Could you check a few things on this model? Use its own coordinates, in mm. Face numbers are marked on the shaded views. A direction names the side the tool comes from. Coordinates: 2 decimals unless noted, no trailing zeros. Loops run counter-clockwise (first coordinate to the right, second up) from the corner with the lowest first, then second, coordinate; pieces in that order, holes last.
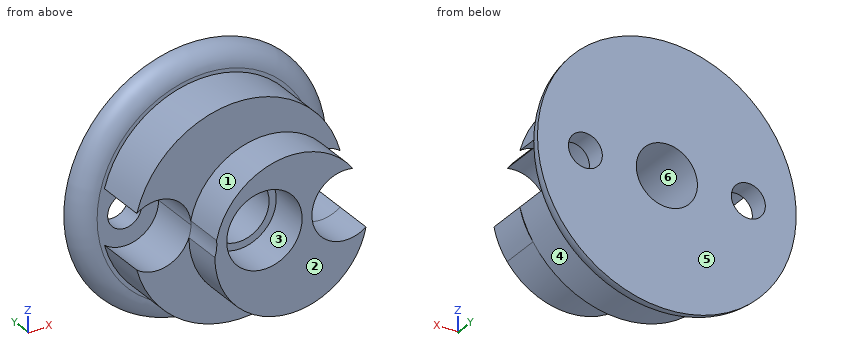
from build123d import *

# Parameters (mm, degrees)
F0_R     = 19.05
F0_R_2   = 2.5
F0_R_3   = 4.5
F1_DEPTH = 3
F2_R     = 2.99999
F3_R     = 4.5
F4_DEPTH = 7.5
F5_R     = 5.555
F6_DEPTH = 6


# Not quite as in the source:
# - a fillet or chamfer is up to 0.001 mm smaller than in the source, because OpenCascade refuses the exact size


with BuildPart() as f1:
    # F0 (on Front) → F1 (new body)
    with BuildSketch(Plane.XZ):
        Circle(F0_R)
        with Locations((-12, 0)):
            Circle(F0_R_2, mode=Mode.SUBTRACT)
        Circle(F0_R_3, mode=Mode.SUBTRACT)
        with Locations((12, 0)):
            Circle(F0_R_2, mode=Mode.SUBTRACT)
    extrude(amount=F1_DEPTH)

    # F2 (radius 3 in the source; OpenCascade refuses exactly that, so slightly less here)
    f2_edges = [f1.edges().sort_by_distance(p)[0] for p in [
        (-19.05, -3, 0),
    ]]
    fillet(f2_edges, radius=F2_R)

    # F3 (on face) → F4 (join)
    with BuildSketch(Plane.XZ.offset(3)):
        with BuildLine():
            ThreePointArc((14.96875, -4.0232478717), (7, 0), (14.96875, 4.0232478717))
            ThreePointArc((14.96875, 4.0232478717), (0, 15.5), (-14.96875, 4.0232478717))
            ThreePointArc((-14.96875, 4.0232478717), (-9.7465304528, 4.4633927678), (-7, 0))
            ThreePointArc((-7, 0), (-9.7465304528, -4.4633927678), (-14.96875, -4.0232478717))
            ThreePointArc((-14.96875, -4.0232478717), (0, -15.5), (14.96875, -4.0232478717))
        make_face()
        Circle(F3_R, mode=Mode.SUBTRACT)
    extrude(amount=F4_DEPTH)

    # F5 (on face) → F6 (join)
    with BuildSketch(Plane.XZ.offset(10.5)):
        with BuildLine():
            ThreePointArc((13.0379586998, -8.3822212416), (14.2369080678, -6.3061863212), (14.96875, -4.0232478717))
            ThreePointArc((14.96875, -4.0232478717), (14.1719474758, -6.2774122648), (13.0379586998, -8.3822212416))
        make_face()
        with BuildLine():
            ThreePointArc((13.0379586998, -8.3822212416), (14.1719474758, -6.2774122648), (14.96875, -4.0232478717))
            ThreePointArc((14.96875, -4.0232478717), (7.1141405648, -1.0622511849), (13.0303045981, 4.8926958249))
            ThreePointArc((13.0303045981, 4.8926958249), (1.6209007027, 9.2560887381), (-7.0415959869, 0.6436067458))
            ThreePointArc((-7.0415959869, 0.6436067458), (-7.0298229821, -0.5452892911), (-7.2990861299, -1.7033522202))
            ThreePointArc((-7.2990861299, -1.7033522202), (0.4406594059, -12.4383718384), (13.0379586998, -8.3822212416))
        make_face()
        Circle(F5_R, mode=Mode.SUBTRACT)
    extrude(amount=F6_DEPTH)


solid = f1.part
1) Imagine slicing it at A-A on y = -10. List the corners of the cut face in (x, z) for me.
2) Imagine slicing it at C-C on y = -1.75. List the corners of the cut face in (x, z) for me.
3) We'd pull the mould along Z, two halves only. Please class the marked faces 4, 5 and 6: released by +Z, released by -Z, zero draft, split by the parting line, or undercut.
4) If I drill on L1, parallel to Y at x = -1, z = -13.5; L2, parallel to Z at x = 12, y = -11.75; L3, parallel to Z at x = 12, y = -0.85, over which ranges is the centre line in solid material (lowest first)?
5) For the marked faces 1, 2 and 3, which set-ups out of +Z, -Z, +X, -X, +Y, -Y let a thin tool reach every point of the face, with its end or its side?
6) Imagine slicing it at D-D on y = -12. List the corners of the cut face in (x, z) for me (3 decimals), plus the area to 3 significant figures.
7) Will these pins go through, and if not, where does the flat tip stop? pin 1 (6 mm diameter, centred on y = -5, z = 8.5, fed in from +X); pin 2 (2 mm diameter, centred on y = -12.5, z = 8.5, fed in from +X); pin 3 (2 mm diameter, centred on y = -2.5, z = 9.5, fed in from -X); pin 4 (4.5 mm diameter, centred on x = 12, z = 0, fed in from +Y).
Solved:
1. outline: (-14.97, -4.02) arc R15.5 ccw to (14.97, -4.02) arc R5 cw (long way) to (14.97, 4.02) arc R15.5 ccw to (-14.97, 4.02) arc R5 cw (long way) to start; hole circle Ø9 at (0, 0)
2. outline: circle Ø36.97 at (0, 0); hole circle Ø5 at (-12, 0); hole circle Ø9 at (0, 0); hole circle Ø5 at (12, 0)
3. face 4: released by -Z
3. face 5: zero draft
3. face 6: undercut
4. L1: y = -10.5 to 0
4. L2: z = -9.61 to -5, 5 to 6.11
4. L3: z = -14.64 to -2.5, 2.5 to 14.64
5. face 1: +Z, -Y
5. face 2: +Z, -Z, +X, -X, -Y
5. face 3: -Y
6. outline: (-7.299, -1.703) arc R11.25 ccw to (14.969, -4.023) arc R5 cw (long way) to (13.03, 4.893) arc R11.25 ccw to (-7.042, 0.644) arc R5 cw to start; hole circle Ø11.11 at (0, 0)
6. area: 235 mm2
7. pin 1: stops at x = 16.5
7. pin 2: stops at x = 10.35
7. pin 3: stops at x = -16.24
7. pin 4: passes through
